Could you check a few things on this model? Use its own coordinates, in mm. Face numbers are marked on the shaded views. A direction names the side the tool comes from. Coordinates: 2 decimals unless noted, no trailing zeros. Write each loop counter-clockwise with the first axis right and the second up, starting at its lowest first coordinate (ties: lowest second). Pieces come first, ordered by that corner, then holes. Notation, with made-up numbers: (-19, 57) - (1, 57) arc R26 cw to (1, 76) - close; hole circle Ø4 at (81.5, 67.25). An arc over 180 degrees is marked (long way). Write item = value, one per line. Start each with the question number.
```python
from build123d import *

# Parameters (mm, degrees)
F1_DEPTH      = 5
F2_DEPTH      = 25
F2_DEPTH_BACK = 25
F3_T1_DEPTH   = 32.333223573
F3_T3_DEPTH   = 16.3059757776
F3_T5_DEPTH   = 2
F3_T7_DEPTH   = 48.4196425394
F3_T9_DEPTH   = 30
F3_T14_DEPTH  = 4.08
F3_T20_DEPTH  = 4.08
F3_T26_DEPTH  = 19.3723096765
F3_T31_DEPTH  = 19.3723096765


# Not quite as in the source:
# - a fillet or chamfer that OpenCascade refuses, or shapes differently, is made with other operations: its cross-section is extruded or revolved along the edge and cut away or added


with BuildPart() as f1:
    # F0 (on Right) → F1 (new body, symmetric)
    with BuildSketch(Plane.YZ):
        Polygon((0, 0), (0, 5), (-8.5454221213, 5), (5.4587286429, 25), (-5.9958492358, 25), (-20, 5), (-20, 0), align=None)
    extrude(amount=F1_DEPTH, both=True)

    # F0 (on Right) → F2 (join, two sides)
    with BuildSketch(Plane.YZ) as f2_sk:
        Polygon((14.0041507642, 25), (0, 5), (0, 0), (50, 0), (25.8219641147, 41.8775865806), align=None)
    extrude(amount=F2_DEPTH)
    extrude(f2_sk.sketch, amount=-F2_DEPTH_BACK)

    # F3: fillet of radius 4 on 8 edges, made by hand

    # F3_s2 → F3_t1 (cut)
    with BuildSketch(Plane(origin=(0, 8.5792437745, 12.2524298959), x_dir=(1, 0, 0), z_dir=(0, -0.5735764364, -0.8191520443))):
        with BuildLine():
            ThreePointArc((-5, 15.2509230675), (-3.8284271247, 18.0793501923), (-1, 19.2509230675))
            Line((-1, 19.2509230675), (-5, 19.2509230675))
            Line((-5, 19.2509230675), (-5, 15.2509230675))
        make_face()
        with BuildLine():
            ThreePointArc((5, 15.2509230675), (3.8284271247, 18.0793501923), (1, 19.2509230675))
            Line((1, 19.2509230675), (5, 19.2509230675))
            Line((5, 19.2509230675), (5, 15.2509230675))
        make_face()
    extrude(amount=F3_T1_DEPTH, mode=Mode.SUBTRACT)

    # F3_s4 → F3_t3 (cut)
    with BuildSketch(Plane.YZ.offset(-8.1529878888)):
        with BuildLine():
            ThreePointArc((-19.2766081772, 6.0331105899), (-19.814867803, 4.9416280425), (-20, 3.7388048445))
            Line((-20, 3.7388048445), (-20, 5))
            Line((-20, 5), (-19.2766081772, 6.0331105899))
        make_face()
    extrude(amount=F3_T3_DEPTH, mode=Mode.SUBTRACT)

    # F3_s6 → F3_t5 (cut)
    with BuildSketch(Plane.YZ.offset(-1)):
        with BuildLine():
            ThreePointArc((-7.1901892108, 23.2943057454), (-5.7605754865, 24.5480433327), (-3.9135810336, 25))
            Line((-3.9135810336, 25), (-5.9958492358, 25))
            Line((-5.9958492358, 25), (-7.1901892108, 23.2943057454))
        make_face()
    extrude(amount=F3_T5_DEPTH, mode=Mode.SUBTRACT)

    # F3_s8 → F3_t7 (cut)
    with BuildSketch(Plane.YZ.offset(-24.2098212697)):
        with BuildLine():
            ThreePointArc((1.0514083121, 18.7056942546), (1.3228434677, 22.8469944529), (-2.225199865, 25))
            Line((-2.225199865, 25), (5.4587286429, 25))
            Line((5.4587286429, 25), (1.0514083121, 18.7056942546))
        make_face()
    extrude(amount=F3_T7_DEPTH, mode=Mode.SUBTRACT)

    # F3_s10 → F3_t9 (cut)
    with BuildSketch(Plane.YZ.offset(-15)):
        with BuildLine():
            ThreePointArc((-16, 0), (-18.8284271247, 1.1715728753), (-20, 4))
            Line((-20, 4), (-20, 0))
            Line((-20, 0), (-16, 0))
        make_face()
    extrude(amount=F3_T9_DEPTH, mode=Mode.SUBTRACT)


with BuildPart() as f3_tool12:
    # F3_s13 → F3_t14 (new body)
    with BuildSketch(Plane.YZ.offset(-1)):
        Polygon((-3.9135810336, 21), (-7.2557213743, 23.3401918603), (-6.0374945998, 25.08), (-3.9135810336, 25.08), align=None)
    extrude(amount=-F3_T14_DEPTH)

    # F3_s15 → F3_t16 (revolve, cut)
    with BuildSketch(Plane(origin=(-1, -3.9135810336, 21), x_dir=(0, 0.4617486132, -0.8870108332), z_dir=(0, 0.8870108332, 0.4617486132))):
        with BuildLine():
            ThreePointArc((0, -4), (4, 0), (0, 4))
            Line((0, 4), (0, -4))
        make_face()
    revolve(axis=Axis((-1, -3.9135810336, 21), (-1, 0, 0)), mode=Mode.SUBTRACT)


with BuildPart() as f1_1:
    add(f1.part)

    # F3_t11: cut F3_tool12
    add(f3_tool12.part, mode=Mode.SUBTRACT)


with BuildPart() as f3_tool18:
    # F3_s19 → F3_t20 (new body)
    with BuildSketch(Plane.YZ.offset(1)):
        Polygon((-3.9135810336, 21), (-7.2557213743, 23.3401918603), (-6.0374945998, 25.08), (-3.9135810336, 25.08), align=None)
    extrude(amount=F3_T20_DEPTH)

    # F3_s21 → F3_t22 (revolve, cut)
    with BuildSketch(Plane(origin=(1, -3.9135810336, 21), x_dir=(0, 0.4617486132, -0.8870108332), z_dir=(0, -0.8870108332, -0.4617486132))):
        with BuildLine():
            ThreePointArc((0, -4), (4, 0), (0, 4))
            Line((0, 4), (0, -4))
        make_face()
    revolve(axis=Axis((1, -3.9135810336, 21), (1, 0, 0)), mode=Mode.SUBTRACT)


with BuildPart() as f1_2:
    add(f1_1.part)

    # F3_t17: cut F3_tool18
    add(f3_tool18.part, mode=Mode.SUBTRACT)


with BuildPart() as f3_tool24:
    # F3_s25 → F3_t26 (new body)
    with BuildSketch(Plane.XZ.offset(-15.4587286429)):
        with BuildLine():
            ThreePointArc((-5, 21), (-3.8284271247, 23.8284271247), (-1, 25))
            Line((-1, 25), (-5, 25))
            Line((-5, 25), (-5, 21))
        make_face()
    extrude(amount=F3_T26_DEPTH)

    split(bisect_by=Plane(origin=(0, -8.083295862, 5.6599846961), x_dir=(1, 0, 0), z_dir=(0, -0.8191520443, 0.5735764364)), keep=Keep.TOP)


with BuildPart() as f1_3:
    add(f1_2.part)

    # F3_t23: cut F3_tool24
    add(f3_tool24.part, mode=Mode.SUBTRACT)


with BuildPart() as f3_tool29:
    # F3_s30 → F3_t31 (new body)
    with BuildSketch(Plane.XZ.offset(-15.4587286429)):
        with BuildLine():
            ThreePointArc((5, 21), (3.8284271247, 23.8284271247), (1, 25))
            Line((1, 25), (5, 25))
            Line((5, 25), (5, 21))
        make_face()
    extrude(amount=F3_T31_DEPTH)

    split(bisect_by=Plane(origin=(0, -8.083295862, 5.6599846961), x_dir=(1, 0, 0), z_dir=(0, -0.8191520443, 0.5735764364)), keep=Keep.TOP)


with BuildPart() as f1_4:
    add(f1_3.part)

    # F3_t28: cut F3_tool29
    add(f3_tool29.part, mode=Mode.SUBTRACT)


solid = f1_4.part
```
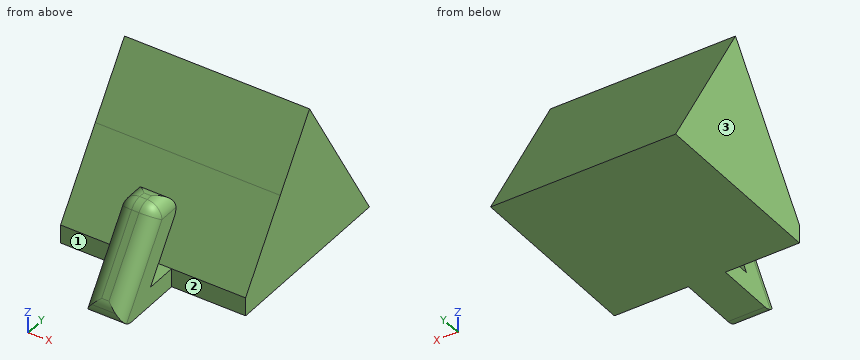
1) Suppose I cut it at A-A on y = -1. Please give me the cut outline in (x, z), plus the area to 3 significant figures.
2) Suppose I cut it at D-D on z = 29.5. Please give me the cut outline in (x, y), plus the area to 3 significant figures.
3) Suppose I cut it at B-B on x = 0. Please give me the cut outline in (y, z).
4) Which directions (+Z, -Z, +X, -X, +Y, -Y) give clear straight access to the entire face, cutting with the end or side of a thin tool? Please do the marked faces 1, 2 and 3.
5) If I drill on probe 1 along Z at (x, y) = (-17.5, 23); probe 2 along Z at (x, y) = (-15.5, 13); probe 3 along Y at (x, z) = (23, 32), over which ranges is the centre line in solid material (lowest first)? Write a range as [from, to].
6) For P1, Ø12, axis at x = 3, z = 32, coming from the -Y side; P2, Ø2.5, axis at x = -13, z = 1.5, coming from the -Y side; P3, Ø10, axis at y = -12.5, z = 11, coming from the +X side, each with a flat end and sliding along its axis, tell me the tip position at first contact or that it passes through.
7) Suppose I cut it at C-C on y = 23. Please give me the cut outline in (x, z), plus the area to 3 significant figures.
Reply:
q1.outline = (-5, 0) - (5, 0) - (5, 5) - (-5, 5) - close; (-5, 15.78) - (5, 15.78) - (5, 21) arc R4 ccw to (2.23, 24.81) - (-2.23, 24.81) arc R4 ccw to (-5, 21) - close
q1.area = 135 mm^2
q2.outline = (-25, 17.16) - (25, 17.16) - (25, 32.97) - (-25, 32.97) - close
q2.area = 791 mm^2
q3.outline = (-20, 3.87) arc R4 ccw to (-16, 0) - (50, 0) - (25.82, 41.88) - (0, 5) - (-8.55, 5) - (1.05, 18.71) arc R4 ccw to (-2.23, 25) - (-3.91, 25) arc R4 ccw to (-7.19, 23.29) - (-19.28, 6.03) arc R4 ccw to start
q4.face_1 = +Z, -Z, -X, -Y
q4.face_2 = +Z, -Z, +X, -Y
q4.face_3 = +Z, -Z, -X, +Y, -Y
q5.probe_1 = [0, 37.85]
q5.probe_2 = [0, 23.57]
q5.probe_3 = [18.91, 31.52]
q6.P1 = 14.7
q6.P2 = 0
q6.P3 = 5
q7.outline = (-25, 0) - (25, 0) - (25, 37.85) - (-25, 37.85) - close
q7.area = 1,890 mm^2
